Can you work these out from the model? Positions are in its coordinate system, mm. Give positions to 0.01 mm unless a question says otherwise; leave off trailing zeros. Write each loop counter-clockwise with the first axis right and the second up, starting at its lowest first coordinate (ties: lowest second). Pieces come first, ordered by that corner, then holes.
1. Suppose I cut it at D-D (y = 27.5). Please give me the cut outline in (x, z).
2. If I drill on probe 1 along Y at (x, z) = (5, 3.2); probe 2 along X at (y, z) = (33.5, 3.55); probe 3 along Y at (x, z) = (98, 0.75), over which ranges is the centre line in solid material (lowest first)?
3. Suppose I cut it at C-C (x = 115). Please give me the cut outline in (y, z).
4. Thinking about a two-plate mould opening in X: for faces 1 (the flat face through (120, 27, 2)), 2 (the cylindrical face through (27.93, 36.016, 2.535)), 3 (the flat face through (59, 28, 5)), which applies, pulls with the +X half, pulls with the -X half, needs draft (parallel to the pull), parting line crosses it, or undercut?
5. I'm going to push a flat-ended pin straight in: pin 1 (3.5 mm diameter, centred on x = 115, y = 50, fed in from +Z). Where does the tip first touch, or does it pass through?
6. Suppose I cut it at B-B (x = 49.5). Please give me the cut outline in (y, z).
7. Suppose I cut it at A-A (y = 50). Please give me the cut outline in (x, z), and give its area (3 significant figures).
```python
from build123d import *

# Parameters (mm, degrees)
F0_W     = 120
F0_H     = 55
F1_DEPTH = 5
F2_R     = 10.1
F3_DEPTH = 5.001
F4_R     = 1.5
F5_DEPTH = 5.001


with BuildPart() as f1:
    # F0 (on Top) → F1 (new body)
    with BuildSketch(Plane.XY):
        with Locations((60, 27.5)):
            Rectangle(F0_W, F0_H)
    extrude(amount=F1_DEPTH)

    # F2 (on face) → F3 (cut, through all)
    with BuildSketch(Plane.XY.offset(5)):
        with Locations((22.5, 27.5)):
            Circle(F2_R)
        with Locations((47.5, 27.5)):
            Circle(F2_R)
        with Locations((72.5, 27.5)):
            Circle(F2_R)
        with Locations((97.5, 27.5)):
            Circle(F2_R)
    extrude(amount=-F3_DEPTH, mode=Mode.SUBTRACT)

    # F4 (on face) → F5 (cut, through all)
    with BuildSketch(Plane.XY.offset(5)):
        with Locations((5, 50)):
            Circle(F4_R)
        with Locations((115, 50)):
            Circle(F4_R)
        with Locations((115, 5)):
            Circle(F4_R)
        with Locations((5, 5)):
            Circle(F4_R)
    extrude(amount=-F5_DEPTH, mode=Mode.SUBTRACT)


solid = f1.part
```
Checks:
1. outline: (0, 0) - (12.4, 0) - (12.4, 5) - (0, 5) - close; (32.6, 0) - (37.4, 0) - (37.4, 5) - (32.6, 5) - close; (57.6, 0) - (62.4, 0) - (62.4, 5) - (57.6, 5) - close; (82.6, 0) - (87.4, 0) - (87.4, 5) - (82.6, 5) - close; (107.6, 0) - (120, 0) - (120, 5) - (107.6, 5) - close
2. probe 1: y = 0 to 3.5, 6.5 to 48.5, 51.5 to 55
2. probe 2: x = 0 to 14.38, 30.62 to 39.38, 55.62 to 64.38, 80.62 to 89.38, 105.62 to 120
2. probe 3: y = 0 to 17.41, 37.59 to 55
3. outline: (0, 0) - (3.5, 0) - (3.5, 5) - (0, 5) - close; (6.5, 0) - (48.5, 0) - (48.5, 5) - (6.5, 5) - close; (51.5, 0) - (55, 0) - (55, 5) - (51.5, 5) - close
4. face 1: pulls with the +X half
4. face 2: undercut
4. face 3: needs draft
5. pin 1: stops at z = 5
6. outline: (0, 0) - (17.6, 0) - (17.6, 5) - (0, 5) - close; (37.4, 0) - (55, 0) - (55, 5) - (37.4, 5) - close
7. outline: (0, 0) - (3.5, 0) - (3.5, 5) - (0, 5) - close; (6.5, 0) - (113.5, 0) - (113.5, 5) - (6.5, 5) - close; (116.5, 0) - (120, 0) - (120, 5) - (116.5, 5) - close
7. area: 570 mm2
